from build123d import *

# Parameters (mm, degrees)
CROQUIS1_R                 = 3
SALIENTE_EXTRUIR2_DEPTH    = 10
CROQUIS2_R                 = 3.51
CORTAR_EXTRUIR1_DEPTH      = 6
CORTAR_EXTRUIR1_DEPTH_BACK = 6
CORTAR_EXTRUIR2_DEPTH      = 13.51


with BuildPart() as part:
    # Croquis1 → Saliente-Extruir2 (new body)
    with BuildSketch(Plane(origin=(0, 0, 0), x_dir=(1, 0, 0), z_dir=(0, 1, 0))):
        with BuildLine():
            ThreePointArc((4.866240612, 7.361217033), (0, 13.51), (-4.866240612, 7.361217033))
            Line((-4.866240612, 7.361217033), (-3.364535629, 1))
            Line((-3.364535629, 1), (3.364535629, 1))
            Line((3.364535629, 1), (4.866240612, 7.361217033))
        make_face()
        with Locations((0, 8.51)):
            Circle(CROQUIS1_R, mode=Mode.SUBTRACT)
    extrude(amount=SALIENTE_EXTRUIR2_DEPTH)

    # Croquis2 → Cortar-Extruir1 (cut, two sides)
    with BuildSketch(Plane(origin=(0, 0, 0), x_dir=(0, 0, -1), z_dir=(1, 0, 0))) as cortar_extruir1_sk:
        with Locations((0, 3.364535629)):
            Circle(CROQUIS2_R)
    extrude(amount=CORTAR_EXTRUIR1_DEPTH, mode=Mode.SUBTRACT)
    extrude(cortar_extruir1_sk.sketch, amount=-CORTAR_EXTRUIR1_DEPTH_BACK, mode=Mode.SUBTRACT)

    # Croquis4 → Cortar-Extruir2 (cut, through all)
    with BuildSketch(Plane.XY.offset(-1)):
        Polygon((-10.381986268, 6.729071258), (12.651385212, 6.729071258), (6.885028009, 11.685095577), (-4.618478965, 12.095500912), align=None)
    extrude(amount=-CORTAR_EXTRUIR2_DEPTH, mode=Mode.SUBTRACT)


solid = part.part
The listing builds one solid part. Answer for the finished solid, in the listing's coordinates (mm). Give positions to 0.01 mm unless a question says otherwise; leave off trailing zeros. Order: outer loops, then holes, each group sorted by start corner. A loop starts at its lowest first (then second) coordinate and runs counter-clockwise, first axis right, second up. Notation, with made-up numbers: (5, 49) - (56, 49) arc R21 ccw to (56, 77) - close; hole circle Ø9 at (83, 17). An arc over 180 degrees is marked (long way). One line per item, written item: value. Start each with the question number.
1) The mould has two halves that part along X. Classify faces 1 (the face through (-2.21, 3.32, -10.54)), 2 (the face through (0.13, 3.32, -13.51)), 3 (the face through (0, 0, -5)): released by +X, released by -X, zero draft, split by the parting line, or undercut.
2) A cutting plane is placed at C-C on y = 3. Give the vertices of the cut face in (x, z), then the cut area to 3 significant figures.
3) A cutting plane is placed at D-D on x = 4.5. Give the vertices of the cut face in (y, z), then the cut area to 3 significant figures.
4) A cutting plane is placed at B-B on x = 0. Give the vertices of the cut face in (y, z), then the cut area to 3 significant figures.
5) Given pin 1 Ø1 at (x, z) = (-1, -10) entering from +Y (1 decimal), flat-ended and moving along its own axis, determine where the tip first touches the part or whether it passes through.
6) Find the intervals of material crossed by L1, parallel to X at y = 2.5, z = -8.51; L2, parallel to Z at x = 0, y = 3.25; L3, parallel to Z at x = -1, y = 3.75, in increasing order.
7) A cutting plane is placed at A-A on z = -8.51. Give the vertices of the cut face in (x, y).
Answer sheet:
1. face 1: undercut
1. face 2: split by the parting line
1. face 3: zero draft
2. outline: (-4.87, -7.36) arc R5 ccw (long way) to (4.87, -7.36) - (3.95, -3.49) - (-3.95, -3.49) - close; hole circle Ø6 at (0, -8.51)
2. area: 56.5 mm2
3. outline: (0, -10.69) - (6.73, -10.69) - (6.73, -5.81) - (0, -5.81) - close
3. area: 32.8 mm2
4. outline: (0, -13.51) - (6.73, -13.51) - (6.73, -11.51) - (0, -11.51) - close; (0, -5.51) - (6.73, -5.51) - (6.73, -1) arc R3.51 cw to (0, -1) - close
4. area: 31.4 mm2
5. pin 1: passes through
6. L1: x = -5 to -3, 3 to 5
6. L2: z = -13.51 to -11.51, -5.51 to -3.51
6. L3: z = -13.41 to -11.34, -5.68 to -3.49
7. outline: (-5, 0) - (-3, 0) - (-3, 6.73) - (-5, 6.73) - close; (3, 0) - (5, 0) - (5, 6.73) - (3, 6.73) - close
